Part model, mm, in its own coordinate system. Face numbers are marked on the shaded views. Give positions to 0.01 mm unless a question says otherwise; leave off trailing zeros.
Autodesk Inventor part; units mm, degrees
ref_plane "YZ Plane" through (0, 0, 0) normal (1, 0, 0) x (0, 1, 0)
ref_plane "XZ Plane" through (0, 0, 0) normal (0, 1, 0) x (-1, 0, 0)
ref_plane "XY Plane" through (0, 0, 0) normal (0, 0, 1) x (1, 0, 0)
sketch "Sketch1" plane through (0, 0, 0) normal (0, 1, 0) x (-1, 0, 0)
  line L0 (0, 1) -> (0, -1)
  line L1 (-4, 1) -> (-4, -1)
  line L2 (-4, -1) -> (-5, -1)
  line L3 (-5, -1) -> (-6.7321, 0)
  line L4 (-6.7321, 0) -> (-5, 1)
  line L5 (-5, 1) -> (-4, 1)
  point P0 (0, 0)
  point P1 (0, 0)
  dimension "d0" = 10
  dimension "d1" = 8
  dimension "d2" = 2
  dimension "d4" = 30
revolve "Revolution1" add sketch "Sketch1" angle 360 about axis through (0, 0, 1) along (0, 0, -1)
sketch "Sketch2" plane through (0, 0, 1) normal (0, 0, 1) x (1, 0, 0)
  circle A0 centre (0, 0) radius 4
  circle A1 centre (0, 0) radius 5
  line L0 (0, 5.7735) -> (5, 2.8868)
  line L1 (5, 2.8868) -> (5, -2.8868)
  line L2 (5, -2.8868) -> (0, -5.7735)
  line L3 (0, -5.7735) -> (-5, -2.8868)
  line L4 (-5, -2.8868) -> (-5, 2.8868)
  line L5 (-5, 2.8868) -> (0, 5.7735)
  point P0 (0, 0)
extrude "Extrusion1" cut sketch "Sketch2" against normal through all keep common part
thread "Thread1"
properties part number "Nut_M8x0.5_2mm" material "Brass, Soft Yellow"
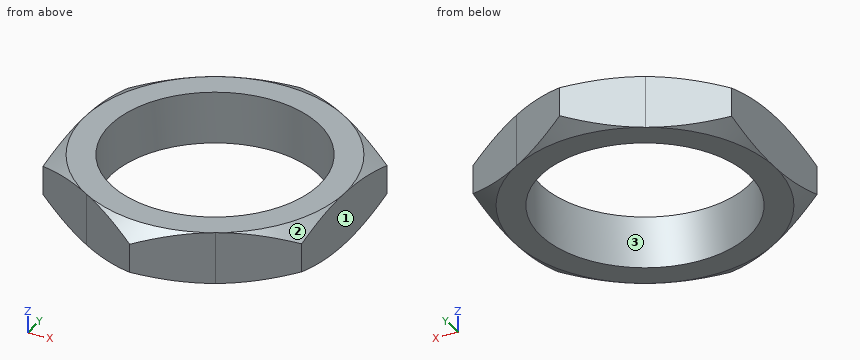
1) Wall check: L1, parallel to X at y = 0, z = -0.1; L2, parallel to Y at x = 0.25, z = 0.3; L3, parallel to Y at x = 1, z = 0.35. Give the ranges that are in metal, low to high.
Answers follow:
L1: x = -5 to -4, 4 to 5
L2: y = -5.63 to -3.99, 3.99 to 5.63
L3: y = -5.2 to -3.87, 3.87 to 5.2
2) Two-plate mould, pull along Y, no slides. Class the marked faces 1, 2 and 3: +Y half, -Y half, draft (parallel to the pull), parting line (faces both ways), or undercut.
Answers follow:
face 1: draft
face 2: -Y half
face 3: undercut
3) Pin check, flat tip, straight feed: pin 1 Ø1 at (y, z) = (-3.5, 1) entering from +X. Stop position of the tip, or through.
Answers follow:
pin 1: stops at x = 4.6
